```python
from build123d import *

# Parameters (mm, degrees)
SFIVEBASETP1_W     = 12.75
SFIVEBASETP1_H     = 13
SFIVEBASETP1_W_2   = 5.5
FFIVEBASETP1_DEPTH = 20


with BuildPart() as part:
    # SFiveBaseTP1 → FFiveBaseTP1 (new body)
    with BuildSketch(Plane(origin=(0, 0, 0), x_dir=(1, 0, 0), z_dir=(0, 1, 0))):
        Polygon((-17.5, 15), (17.5, 15), (17.5, 0), (7.5, -17.320508076), (-7.5, -17.320508076), (-17.5, 0), align=None)
        Polygon((-16.345299462, 0), (-6.922649731, -16.320508076), (-0.5, -16.320508076), (-0.5, 0), align=None, mode=Mode.SUBTRACT)
        with Locations((-10.125, 7.5)):
            Rectangle(SFIVEBASETP1_W, SFIVEBASETP1_H, mode=Mode.SUBTRACT)
        with Locations((10.125, 7.5)):
            Rectangle(SFIVEBASETP1_W, SFIVEBASETP1_H, mode=Mode.SUBTRACT)
        Polygon((0.5, 0), (0.5, -16.320508076), (6.922649731, -16.320508076), (16.345299462, 0), align=None, mode=Mode.SUBTRACT)
        with Locations((0, 7.5)):
            Rectangle(SFIVEBASETP1_W_2, SFIVEBASETP1_H, mode=Mode.SUBTRACT)
    extrude(amount=FFIVEBASETP1_DEPTH)


solid = part.part
```
Could you check a few things on this model? Use its own coordinates, in mm. A direction names the side the tool comes from. Coordinates: 2 decimals unless noted, no trailing zeros. Write each loop counter-clockwise with the first axis right and the second up, starting at its lowest first coordinate (ties: lowest second). Pieces come first, ordered by that corner, then holes. Notation, with made-up numbers: (-38, -35.75) -> (11, -35.75) arc R20 cw to (11, -17.75) -> close; hole circle Ø1 at (65.25, -21.5). An arc over 180 degrees is marked (long way). One line per question, with ' | ' between items. Start each with the question number.
1. If we section it at B-B (x = -5): Please give me the cut outline in (y, z).
2. Thinking about a two-plate mould opening in X: for faces 1 (the face through (-12.43, 9.86, 8.78)), 2 (the face through (11.57, 9.86, 8.27)), 3 (the face through (0, 10, 17.321)), which applies, pulls with the +X half, pulls with the -X half, needs draft (parallel to the pull), parting line crosses it, or undercut?
3. If we section it at A-A (z = -6): Please give me the cut outline in (x, y).
4. Please list where these lines run through material, in increasing order: line 1 along Z through (x, y) = (-2, 11.75); line 2 along X through (y, z) = (14.5, -4); line 3 along Z through (x, y) = (-8.5, 18.25).
5. If we section it at C-C (y = 2): Please give me the cut outline in (x, z).
6. Will these pins go through, and if not, where does the flat tip stop? P1, Ø5, axis at y = 7.5, z = 9, coming from the +X side; P2, Ø5, axis at y = 10.5, z = 5, coming from the -X side; P3, Ø1, axis at y = 14.5, z = 10, coming from the +X side.
7. For faces 4 (the face through (0, 20, 1)), 5 (the face through (10, 10, -14)), which set-ups out of +Z, -Z, +X, -X, +Y, -Y let a thin tool reach every point of the face, with its end or its side?
8. If we section it at D-D (z = 3): Please give me the cut outline in (x, y).
Return value:
1) outline: (0, -15) -> (20, -15) -> (20, -14) -> (0, -14) -> close; (0, -1) -> (20, -1) -> (20, 0) -> (0, 0) -> close; (0, 16.32) -> (20, 16.32) -> (20, 17.32) -> (0, 17.32) -> close
2) face 1: pulls with the -X half | face 2: undercut | face 3: needs draft
3) outline: (-17.5, 0) -> (-16.5, 0) -> (-16.5, 20) -> (-17.5, 20) -> close; (-3.75, 0) -> (-2.75, 0) -> (-2.75, 20) -> (-3.75, 20) -> close; (2.75, 0) -> (3.75, 0) -> (3.75, 20) -> (2.75, 20) -> close; (16.5, 0) -> (17.5, 0) -> (17.5, 20) -> (16.5, 20) -> close
4) line 1: z = -15 to -14, -1 to 0, 16.32 to 17.32 | line 2: x = -17.5 to -16.5, -3.75 to -2.75, 2.75 to 3.75, 16.5 to 17.5 | line 3: z = -15 to -14, -1 to 0, 13.59 to 15.59
5) outline: (-17.5, -15) -> (17.5, -15) -> (17.5, 0) -> (7.5, 17.32) -> (-7.5, 17.32) -> (-17.5, 0) -> close; hole (-16.5, -14) -> (-3.75, -14) -> (-3.75, -1) -> (-16.5, -1) -> close; hole (-16.35, 0) -> (-0.5, 0) -> (-0.5, 16.32) -> (-6.92, 16.32) -> close; hole (-2.75, -14) -> (2.75, -14) -> (2.75, -1) -> (-2.75, -1) -> close; hole (0.5, 0) -> (16.35, 0) -> (6.92, 16.32) -> (0.5, 16.32) -> close; hole (3.75, -14) -> (16.5, -14) -> (16.5, -1) -> (3.75, -1) -> close
6) P1: stops at x = 13.75 | P2: stops at x = -16.06 | P3: stops at x = 12.02
7) face 4: +Z, -Z, +X, -X, +Y | face 5: +Y, -Y
8) outline: (-15.77, 0) -> (-14.61, 0) -> (-14.61, 20) -> (-15.77, 20) -> close; (-0.5, 0) -> (0.5, 0) -> (0.5, 20) -> (-0.5, 20) -> close; (14.61, 0) -> (15.77, 0) -> (15.77, 20) -> (14.61, 20) -> close
